from build123d import *

# Parameters (mm, degrees)
SKETCH1_R           = 5
BOSS_EXTRUDE1_DEPTH = 60
CUT_EXTRUDE1_DEPTH  = 55
CUT_EXTRUDE2_DEPTH  = 3.5
FILLET1_R           = 3
SKETCH4_W           = 18
SKETCH4_H           = 20
CUT_EXTRUDE3_DEPTH  = 3.5
FILLET3_R           = 7
FILLET4_R           = 1
FILLET5_R           = 8
FILLET6_R           = 5


with BuildPart() as part:
    # Sketch1 → Boss-Extrude1 (new body)
    # profile 1 of 2: a face of its own
    with BuildSketch(Plane.XY):
        with BuildLine():
            ThreePointArc((-201.458607688, 71.281187739), (-127.708935748, -35.593764587), (-4.542381846, -76.718812261))
            Line((-4.542381846, -76.718812261), (-4.542381846, -6.718812261))
            Line((-4.542381846, -6.718812261), (-4.542381846, 13.281187739))
            Line((-4.542381846, 13.281187739), (-44.542381846, 13.281187739))
            Line((-44.542381846, 13.281187739), (-44.542381846, 56.281187739))
            Line((-44.542381846, 56.281187739), (-64.242381846, 56.281187739))
            Line((-64.242381846, 56.281187739), (-64.242381846, 16.281187739))
            Line((-64.242381846, 16.281187739), (-67.842381846, 16.281187739))
            Line((-67.842381846, 16.281187739), (-67.842381846, 56.281187739))
            Line((-67.842381846, 56.281187739), (-87.542381846, 56.281187739))
            Line((-87.542381846, 56.281187739), (-87.542381846, 71.281187739))
            Line((-87.542381846, 71.281187739), (-201.458607688, 71.281187739))
        make_face()
        with Locations((-177.542381846, 49.281187739)):
            Circle(SKETCH1_R, mode=Mode.SUBTRACT)
    # profile 2 of 2: a face of its own
    with BuildSketch(Plane.XY):
        with BuildLine():
            Line((-4.542381846, -80.718812261), (-4.542381846, -76.718812261))
            ThreePointArc((-4.542381846, -76.718812261), (-127.708935748, -35.593764587), (-201.458607688, 71.281187739))
            Line((-201.458607688, 71.281187739), (-205.405610163, 71.281187739))
            ThreePointArc((-205.405610163, 71.281187739), (-130.035471154, -37.836764924), (-4.542381846, -80.718812261))
        make_face()
    extrude(amount=BOSS_EXTRUDE1_DEPTH)

    # Sketch2 → Cut-Extrude1 (cut)
    with BuildSketch(Plane.XY.offset(60)):
        with BuildLine():
            Line((-4.542381846, 71.281187739), (-4.542381846, -76.718812261))
            ThreePointArc((-4.542381846, -76.718812261), (-127.708935748, -35.593764587), (-201.458607688, 71.281187739))
            Line((-201.458607688, 71.281187739), (-4.542381846, 71.281187739))
        make_face()
    extrude(amount=-CUT_EXTRUDE1_DEPTH, mode=Mode.SUBTRACT)

    # Sketch3 → Cut-Extrude2 (cut)
    with BuildSketch(Plane(origin=(0, 0, 0), x_dir=(-1, 0, 0), z_dir=(0, 0, -1))):
        Polygon((4.542381846, -61.718812261), (49.542381846, -61.718812261), (49.542381846, -51.718812261), (49.542381846, -21.718812261), (49.542381846, -1.718812261), (4.542381846, -1.718812261), (4.542381846, -11.718812261), (39.542381846, -11.718812261), (39.542381846, -51.718812261), (4.542381846, -51.718812261), align=None)
    extrude(amount=-CUT_EXTRUDE2_DEPTH, mode=Mode.SUBTRACT)

    # Fillet1
    fillet1_edges = [part.edges().sort_by_distance(p)[0] for p in [
        (-130.035471154, -37.836764924, 60),
        (-130.035471154, -37.836764924, 0),
    ]]
    fillet(fillet1_edges, radius=FILLET1_R)

    # Sketch4 → Cut-Extrude3 (cut)
    with BuildSketch(Plane(origin=(0, 0, 0), x_dir=(-1, 0, 0), z_dir=(0, 0, -1))):
        Polygon((102.842381846, -4.039320336), (134.019296382, 13.960679664), (124.019296382, 31.281187739), (92.842381846, 13.281187739), align=None)
        with Locations((13.542381846, -31.718812261)):
            Rectangle(SKETCH4_W, SKETCH4_H)
    extrude(amount=-CUT_EXTRUDE3_DEPTH, mode=Mode.SUBTRACT)

    # Fillet3
    fillet3_edges = [part.edges().sort_by_distance(p)[0] for p in [
        (-102.842381846, -4.039320336, 1.75),
        (-92.842381846, 13.281187739, 1.75),
        (-124.019296382, 31.281187739, 1.75),
        (-134.019296382, 13.960679664, 1.75),
        (-22.542381846, -21.718812261, 1.75),
        (-22.542381846, -41.718812261, 1.75),
    ]]
    fillet(fillet3_edges, radius=FILLET3_R)

    # Fillet4
    fillet4_edges = [part.edges().sort_by_distance(p)[0] for p in [
        (-87.542381846, 56.281187739, 2.5),
        (-44.542381846, 13.281187739, 2.5),
    ]]
    fillet(fillet4_edges, radius=FILLET4_R)

    # Fillet5
    fillet5_edges = [part.edges().sort_by_distance(p)[0] for p in [
        (-49.542381846, -1.718812261, 1.75),
        (-49.542381846, -61.718812261, 1.75),
    ]]
    fillet(fillet5_edges, radius=FILLET5_R)

    # Fillet6
    fillet6_edges = [part.edges().sort_by_distance(p)[0] for p in [
        (-39.542381846, -51.718812261, 1.75),
        (-39.542381846, -11.718812261, 1.75),
    ]]
    fillet(fillet6_edges, radius=FILLET6_R)


solid = part.part
The listing builds one solid part. Answer for the finished solid, in the listing's coordinates (mm). A direction names the side the tool comes from. Coordinates: 2 decimals unless noted, no trailing zeros. Loops run counter-clockwise (first coordinate to the right, second up) from the corner with the lowest first, then second, coordinate; pieces in that order, holes last. Notation, with made-up numbers: (38.25, -12) -> (70.25, -12) arc R29 cw to (70.25, 27) -> close; hole circle Ø9 at (13, 37.5). An arc over 180 degrees is marked (long way). Write item = value, one per line. Start each with the question number.
1) Straight lines are drawn through the part: line 1 (Z direction, x = -20, y = -4); line 2 (Z direction, x = -176, y = 62); line 3 (X direction, y = -26, z = 54). For each, find the intervals that lie inside material, in ascending order. Write a range as from..to.
2) The mould has two halves that part along X. Classify faces 4 (the face through (-77, 56.281, 2)), 5 (the face through (-38.039, -13.145, 1.774)), 6 (the face through (-20.437, -23.715, 1.774)): released by +X, released by -X, zero draft, split by the parting line, or undercut.
3) A tool of negligible diameter and unlimited length cuts with its end or side. For faces 1 (the face through (-24, 13.281, 2)), 2 (the face through (-20.44, -39.72, 1.77)), 3 (the face through (-64.242, 37, 2)), from which of +Z, -Z, +X, -X, +Y, -Y can it reach the whole face along a straight path? Write none if from no direction.
4) Given pin 1 Ø12 at (x, z) = (-38, 8.5) entering from -Y; pin 2 Ø1.8 at (y, z) = (-33, 2.5) entering from +X; pin 3 Ø5.5 at (y, z) = (67, 3) entering from +X; pin 4 Ø6 at (x, y) = (-173.5, 36.5) entering from -Z, each flat-ended and moving along its own axis, determine where each tip first touches the part or whether it passes through.
5) A cutting plane is placed at A-A (z = 21.5). Give the vertices of the cut face in (x, y), then the cut area to 3 significant figures.
Responses:
q1.line_1 = 3.5..5
q1.line_2 = 0..5
q1.line_3 = -144.33..-139.53
q2.face_4 = zero draft
q2.face_5 = undercut
q2.face_6 = released by +X
q3.face_1 = +Z, -Z, +X, +Y
q3.face_2 = -Z, +X
q3.face_3 = +Z, -Z, +Y
q4.pin_1 = -78.63
q4.pin_2 = -22.54
q4.pin_3 = -87.54
q4.pin_4 = 0
q5.outline = (-205.41, 71.28) arc R211.73 ccw to (-4.54, -80.72) -> (-4.54, -76.72) arc R205 cw to (-201.46, 71.28) -> close
q5.area = 916 mm²
